Geometry: final body of the model. Coordinates: model frame, mm. Face numbers are marked on the shaded views. A direction names the side the tool comes from. Give positions to 0.01 mm unless a question says otherwise; leave off trailing zeros. Loops run counter-clockwise (first coordinate to the right, second up) from the corner with the lowest first, then second, coordinate; pieces in that order, holes last.
1. Material intervals for line 1 along X through (y, z) = (51, -2); line 2 along Y through (x, z) = (104.6, 52.35); line 3 along Y through (x, z) = (85, -2.7), sorted ascending.
2. Section C-C, the plane z = 35. Output: boundary loops of the cut face in (x, y).
3. Section A-A, the plane y = 12.5. Output: boundary loops of the cut face in (x, z).
4. Draft query along X for the marked faces 1, 2 and 3. Return one class per face: +X half, -X half, draft (parallel to the pull), parting line (faces both ways), or undercut.
5. Section B-B, the plane x = 85. Output: boundary loops of the cut face in (y, z), then the cut area to 3 significant figures.
6. First-contact query: P1, Ø1.5, axis at x = 66, y = 30.5, coming from the +Z side; P2, Ø2, axis at y = 3.5, z = 50, coming from the -X side. Flat tips, straight axial feed; report the tip coordinate or a pass-through.
7. Access query for the marked faces 4 and 5. Directions: +Z, -Z, +X, -X, +Y, -Y. A direction counts if a zero-diameter tool reaches every point of the face in a straight line with its end or side. Return the directions, or none.
8. Section D-D, the plane x = 99.5. Output: boundary loops of the cut face in (y, z), then the cut area to 3 significant figures.
from build123d import *

# Parameters (mm, degrees)
SKETCH1_W           = 107.6
SKETCH1_H           = 59.3
SKETCH1_W_2         = 103.6
SKETCH1_H_2         = 55.3
BOSS_EXTRUDE1_DEPTH = 55
SKETCH2_W           = 107.6
SKETCH2_H           = 59.3
SKETCH2_R           = 1.5
BOSS_EXTRUDE2_DEPTH = 3
SKETCH3_R           = 2.5
CUT_EXTRUDE1_DEPTH  = 1.5
SKETCH4_W           = 12
SKETCH4_H           = 10
CUT_EXTRUDE2_DEPTH  = 5
SKETCH5_W           = 35
SKETCH5_H           = 5
CUT_EXTRUDE3_DEPTH  = 5
SKETCH8_R           = 1.75
CUT_EXTRUDE4_DEPTH  = 10
CHAMFER1_SIZE       = 2
SKETCH9_W           = 4
SKETCH9_H           = 4
BOSS_EXTRUDE4_DEPTH = 8
CHAMFER2_SIZE       = 4
SKETCH10_R          = 1.25
CUT_EXTRUDE5_DEPTH  = 5


with BuildPart() as part:
    # Sketch1 → Boss-Extrude1 (new body)
    with BuildSketch(Plane.XY):
        with Locations((53.8, 29.65)):
            Rectangle(SKETCH1_W, SKETCH1_H)
        with Locations((53.8, 29.65)):
            Rectangle(SKETCH1_W_2, SKETCH1_H_2, mode=Mode.SUBTRACT)
    extrude(amount=BOSS_EXTRUDE1_DEPTH)

    # Sketch2 → Boss-Extrude2 (add)
    with BuildSketch(Plane(origin=(0, 0, 0), x_dir=(-1, 0, 0), z_dir=(0, 0, -1))):
        with Locations((-53.8, 29.65)):
            Rectangle(SKETCH2_W, SKETCH2_H)
        with Locations((-18.3, 53.7)):
            Circle(SKETCH2_R, mode=Mode.SUBTRACT)
        with Locations((-17, 5.5)):
            Circle(SKETCH2_R, mode=Mode.SUBTRACT)
        with Locations((-93.2, 53.7)):
            Circle(SKETCH2_R, mode=Mode.SUBTRACT)
        with Locations((-99.5, 5.5)):
            Circle(SKETCH2_R, mode=Mode.SUBTRACT)
    extrude(amount=BOSS_EXTRUDE2_DEPTH)

    # Sketch3 → Cut-Extrude1 (cut)
    with BuildSketch(Plane(origin=(0, 0, -3), x_dir=(-1, 0, 0), z_dir=(0, 0, -1))):
        with Locations((-93.2, 53.7)):
            Circle(SKETCH3_R)
        with Locations((-18.3, 53.7)):
            Circle(SKETCH3_R)
        with Locations((-17, 5.5)):
            Circle(SKETCH3_R)
        with Locations((-99.5, 5.5)):
            Circle(SKETCH3_R)
    extrude(amount=-CUT_EXTRUDE1_DEPTH, mode=Mode.SUBTRACT)

    # Sketch4 → Cut-Extrude2 (cut)
    with BuildSketch(Plane.ZY):
        with Locations((17, 11.5)):
            Rectangle(SKETCH4_W, SKETCH4_H)
    extrude(amount=-CUT_EXTRUDE2_DEPTH, mode=Mode.SUBTRACT)

    # Sketch5 → Cut-Extrude3 (cut)
    with BuildSketch(Plane(origin=(107.6, 0, 0), x_dir=(0, 0, -1), z_dir=(1, 0, 0))):
        with Locations((-37.5, 38)):
            Rectangle(SKETCH5_W, SKETCH5_H)
    extrude(amount=-CUT_EXTRUDE3_DEPTH, mode=Mode.SUBTRACT)

    # Sketch8 → Cut-Extrude4 (cut)
    with BuildSketch(Plane.XY):
        with Locations((10, 51.3)):
            Circle(SKETCH8_R)
        with Locations((85, 51.3)):
            Circle(SKETCH8_R)
        with Locations((85, 7.3)):
            Circle(SKETCH8_R)
        with Locations((10, 7.3)):
            Circle(SKETCH8_R)
    extrude(amount=-CUT_EXTRUDE4_DEPTH, mode=Mode.SUBTRACT)

    # Chamfer1
    chamfer1_edges = [part.edges().sort_by_distance(p)[0] for p in [
        (8.25, 7.3, 0),
        (83.25, 7.3, 0),
        (83.25, 51.3, 0),
        (8.25, 51.3, 0),
    ]]
    chamfer(chamfer1_edges, length=CHAMFER1_SIZE)

    # Sketch9 → Boss-Extrude4 (add)
    with BuildSketch(Plane.XY.offset(55)):
        with Locations((4, 4)):
            Rectangle(SKETCH9_W, SKETCH9_H)
        with Locations((103.6, 55.3)):
            Rectangle(SKETCH9_W, SKETCH9_H)
        with Locations((103.6, 4)):
            Rectangle(SKETCH9_W, SKETCH9_H)
        with Locations((4, 55.3)):
            Rectangle(SKETCH9_W, SKETCH9_H)
    extrude(amount=-BOSS_EXTRUDE4_DEPTH)

    # Chamfer2
    chamfer2_edges = [part.edges().sort_by_distance(p)[0] for p in [
        (4, 57.3, 47),
        (2, 55.3, 47),
        (4, 2, 47),
        (2, 4, 47),
        (105.6, 4, 47),
        (103.6, 2, 47),
        (103.6, 57.3, 47),
        (105.6, 55.3, 47),
    ]]
    chamfer(chamfer2_edges, length=CHAMFER2_SIZE - 0.0001)  # a hair under: the kernel refuses the full size

    # Sketch10 → Cut-Extrude5 (cut)
    with BuildSketch(Plane.XY.offset(55)):
        with Locations((3, 56.3)):
            Circle(SKETCH10_R)
        with Locations((104.6, 56.3)):
            Circle(SKETCH10_R)
        with Locations((104.6, 3)):
            Circle(SKETCH10_R)
        with Locations((3, 3)):
            Circle(SKETCH10_R)
    extrude(amount=-CUT_EXTRUDE5_DEPTH, mode=Mode.SUBTRACT)


solid = part.part
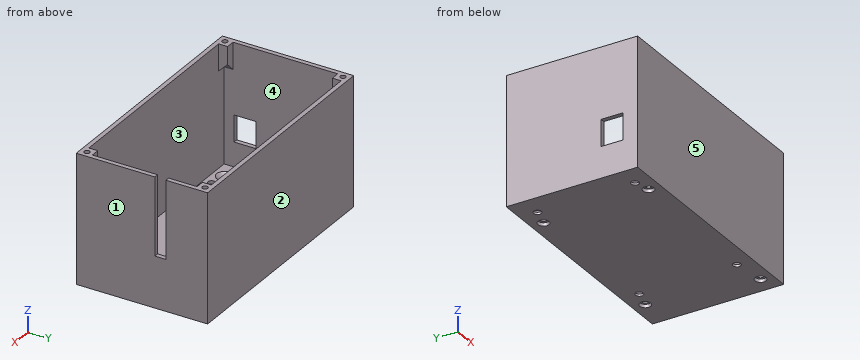
Answers below:
1. line 1: x = 0 to 8.28, 11.72 to 83.28, 86.72 to 107.6
1. line 2: y = 0 to 1.75, 4.25 to 6, 53.3 to 55.05, 57.55 to 59.3
1. line 3: y = 0 to 5.55, 9.05 to 49.55, 53.05 to 59.3
2. outline: (0, 0) - (107.6, 0) - (107.6, 35.5) - (105.6, 35.5) - (105.6, 2) - (2, 2) - (2, 57.3) - (105.6, 57.3) - (105.6, 40.5) - (107.6, 40.5) - (107.6, 59.3) - (0, 59.3) - close
3. outline: (0, -3) - (107.6, -3) - (107.6, 55) - (105.6, 55) - (105.6, 0) - (2, 0) - (2, 11) - (0, 11) - close; (0, 23) - (2, 23) - (2, 55) - (0, 55) - close
4. face 1: +X half
4. face 2: draft
4. face 3: undercut
5. outline: (0, -3) - (5.55, -3) - (5.55, -2) - (3.55, 0) - (2, 0) - (2, 55) - (0, 55) - close; (9.05, -3) - (49.55, -3) - (49.55, -2) - (47.55, 0) - (11.05, 0) - (9.05, -2) - close; (53.05, -3) - (59.3, -3) - (59.3, 55) - (57.3, 55) - (57.3, 0) - (55.05, 0) - (53.05, -2) - close
5. area: 369 mm2
6. P1: stops at z = 0
6. P2: stops at x = 0
7. face 4: none
7. face 5: +Z, -Z, +X, -X, -Y
8. outline: (0, -3) - (3, -3) - (3, -1.5) - (4, -1.5) - (4, 0) - (2, 0) - (2, 55) - (0, 55) - close; (7, -1.5) - (8, -1.5) - (8, -3) - (59.3, -3) - (59.3, 55) - (57.3, 55) - (57.3, 0) - (7, 0) - close
8. area: 386 mm2
